```python
from build123d import *

# Parameters (mm, degrees)
BOSS_EXTRUDE1_DEPTH       = 5
M3X0_5_TAPPED_HOLE1_D     = 2.5
M3X0_5_TAPPED_HOLE1_DEPTH = 7.5
M3X0_5_TAPPED_HOLE1_TIP   = 0.751075774
M3X0_5_TAPPED_HOLE2_D     = 2.5
M3X0_5_TAPPED_HOLE2_DEPTH = 7.5
M3X0_5_TAPPED_HOLE2_TIP   = 0.751075774
M3X0_5_TAPPED_HOLE3_D     = 2.5
M3X0_5_TAPPED_HOLE3_DEPTH = 7.5
M3X0_5_TAPPED_HOLE3_TIP   = 0.751075774
M3X0_5_TAPPED_HOLE4_D     = 2.5
M3X0_5_TAPPED_HOLE4_DEPTH = 7.5
M3X0_5_TAPPED_HOLE4_TIP   = 0.751075774


with BuildPart() as part:
    # Sketch1 → Boss-Extrude1 (new body)
    with BuildSketch(Plane(origin=(0, 0, 0), x_dir=(1, 0, 0), z_dir=(0, 1, 0))):
        Polygon((0, -39), (75, -80), (75, 0), (0, 0), align=None)
    extrude(amount=-BOSS_EXTRUDE1_DEPTH)

    # M3x0.5 Tapped Hole1
    with Locations(Plane(origin=(0, 0, 0), x_dir=(-1, 0, 0), z_dir=(0, 0, -1))):
        with Locations((-15, -2.5), (-60, -2.5)):
            Hole(M3X0_5_TAPPED_HOLE1_D / 2, depth=M3X0_5_TAPPED_HOLE1_DEPTH)
            with Locations((0, 0, -(M3X0_5_TAPPED_HOLE1_DEPTH + M3X0_5_TAPPED_HOLE1_TIP / 2))):  # 118° drill point
                Cone(0, M3X0_5_TAPPED_HOLE1_D / 2, M3X0_5_TAPPED_HOLE1_TIP, mode=Mode.SUBTRACT)

    # M3x0.5 Tapped Hole2
    with Locations(Plane.ZY):
        with Locations((10, -2.5), (25, -2.5)):
            Hole(M3X0_5_TAPPED_HOLE2_D / 2, depth=M3X0_5_TAPPED_HOLE2_DEPTH)
            with Locations((0, 0, -(M3X0_5_TAPPED_HOLE2_DEPTH + M3X0_5_TAPPED_HOLE2_TIP / 2))):  # 118° drill point
                Cone(0, M3X0_5_TAPPED_HOLE2_D / 2, M3X0_5_TAPPED_HOLE2_TIP, mode=Mode.SUBTRACT)

    # M3x0.5 Tapped Hole3
    with Locations(Plane(origin=(75, 0, 0), x_dir=(0, 0, -1), z_dir=(1, 0, 0))):
        with Locations((-20, -2.5), (-60, -2.5)):
            Hole(M3X0_5_TAPPED_HOLE3_D / 2, depth=M3X0_5_TAPPED_HOLE3_DEPTH)
            with Locations((0, 0, -(M3X0_5_TAPPED_HOLE3_DEPTH + M3X0_5_TAPPED_HOLE3_TIP / 2))):  # 118° drill point
                Cone(0, M3X0_5_TAPPED_HOLE3_D / 2, M3X0_5_TAPPED_HOLE3_TIP, mode=Mode.SUBTRACT)

    # M3x0.5 Tapped Hole4
    with Locations(Plane(origin=(-16.414590747, 0, 30.026690391), x_dir=(0.8774480829328538, 0, 0.4796716186699602), z_dir=(-0.4796716186699602, 0, 0.8774480829328538))):
        with Locations((44.182335714, -2.5), (84.182335714, -2.5)):
            Hole(M3X0_5_TAPPED_HOLE4_D / 2, depth=M3X0_5_TAPPED_HOLE4_DEPTH)
            with Locations((0, 0, -(M3X0_5_TAPPED_HOLE4_DEPTH + M3X0_5_TAPPED_HOLE4_TIP / 2))):  # 118° drill point
                Cone(0, M3X0_5_TAPPED_HOLE4_D / 2, M3X0_5_TAPPED_HOLE4_TIP, mode=Mode.SUBTRACT)


solid = part.part
```
Part model, mm, in its own coordinate system. A direction names the side the tool comes from. Give positions to 0.01 mm unless a question says otherwise; leave off trailing zeros. Order: outer loops, then holes, each group sorted by start corner. A loop starts at its lowest first (then second) coordinate and runs counter-clockwise, first axis right, second up. Notation, with made-up numbers: M 78,-3 L 125,-3 A38 ccw 125,35 Z; hole C 44,-18.75 d10. An arc over 180 degrees is marked long. Use a Markdown table: item, result. Add a question column.
(1) 3-axis set-ups, long thin cutter, end or side, ignore diameter. For faces 1 (the face through (71.2, -2.12, 61.19)), 2 (the face through (58.23, -2.12, 66.5)), 3 (the face through (3.8, -2.45, 11.25)), 4 (the face through (14.079, -1.655, 3.802)), 5 (the face through (38, -2, 0)): which of +Z, -Z, +X, -X, +Y, -Y reach the whole face in a straight line?
(2) Saw through at A-A, the plane x = 37.5. Give the cut face in (y, z).
(3) Saw through at B-B, the plane x = 30. Give the cut face in (y, z), and give its area (3 significant figures).
(4) Probe line 1 along X through (y, z) = (-2.5, 2.75); line 2 along Y through (x, z) = (2, 10); line 3 along Z through (x, y) = (71.5, -2.5). List the from-to ranges inside material, lowest first. Write a range as [from, to].
(5) Drop flat-ended pins along their axis: P1, Ø1.5, axis at y = -0.5, z = 56.5, coming from the -X side; P2, Ø2, axis at y = -2.5, z = 60, coming from the -X side; P3, Ø2, axis at y = -2.5, z = 20, coming from the +X side. Give the stop position or say it passes through.
(6) Mould opens along X. For faces 6 (the face through (0, -2, 19)), 7 (the face through (61.19, -2.12, 3.8)), 8 (the face through (61.522, -2.583, 63.377)), 9 (the face through (37, 0, 31)) say: +X half, -X half, draft (parallel to the pull), parting line (faces both ways), or undercut.
Answer key:
| question | item | result |
|---|---|---|
| 1 | face 1 | +X |
| 1 | face 2 | none |
| 1 | face 3 | -X |
| 1 | face 4 | -Z |
| 1 | face 5 | -Z, +X, -X, +Y, -Y |
| 2 | outline | M -5,0 L 0,0 L 0,59.5 L -5,59.5 Z |
| 3 | outline | M -5,0 L 0,0 L 0,55.4 L -5,55.4 Z |
| 3 | area | 277 mm^2 |
| 4 | line 1 | [0, 13.75], [16.25, 58.75], [61.25, 75] |
| 4 | line 2 | [-5, -3.75], [-1.25, 0] |
| 4 | line 3 | [0, 18.75], [21.25, 58.75], [61.25, 78.09] |
| 5 | P1 | x = 30.64 |
| 5 | P2 | x = 36.59 |
| 5 | P3 | x = 67.35 |
| 6 | face 6 | -X half |
| 6 | face 7 | undercut |
| 6 | face 8 | undercut |
| 6 | face 9 | draft |
